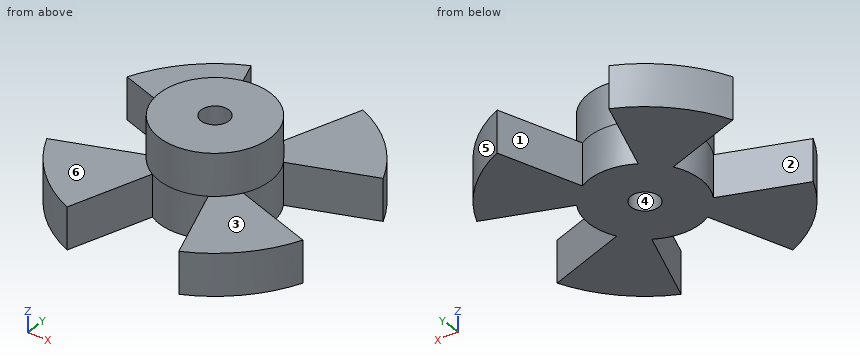
Autodesk Inventor part; units mm, degrees
ref_plane "YZ Plane" through (0, 0, 0) normal (1, 0, 0) x (0, 1, 0)
ref_plane "XZ Plane" through (0, 0, 0) normal (0, 1, 0) x (-1, 0, 0)
ref_plane "XY Plane" through (0, 0, 0) normal (0, 0, 1) x (1, 0, 0)
sketch "Esquisse1" plane through (0, 0, 0) normal (0, 0, 1) x (1, 0, 0)
  circle A0 centre (0, 0) radius 5
  dimension "d0" = 10
extrude "Extrusion1" add sketch "Esquisse1" along normal blind 1.5
sketch "Esquisse2" plane through (0, 0, 1.5) normal (0, 0, 1) x (1, 0, 0)
  circle A0 centre (0, 0) radius 5
  circle A1 centre (0, 0) radius 2
  dimension "d3" = 4
extrude "Extrusion2" add sketch "Esquisse2" along normal blind 1.5 contours A1
sketch "Esquisse3" plane through (0, 0, 1.5) normal (0, 0, 1) x (1, 0, 0)
  circle A0 centre (0, 0) radius 2
  circle A1 centre (0, 0) radius 5
  line L0 (-2, 4.5826) -> (-1, 1.7321)
  line L1 (1, 1.7321) -> (2, 4.5826)
  arc A2 (1, 1.7321) -> (-1, 1.7321) centre (0, 0) ccw
  arc A3 (2, 4.5826) -> (-2, 4.5826) centre (0, 0) ccw
extrude "Extrusion3" cut sketch "Esquisse3" against normal through all contours A0 L0 A1 L1 picked at (1.2132, 3.7931)
pattern_circular "Réseau circulaire1" count 4 over 360 about axis through (0, 0, 1.5) along (0, 0, 1) of "Extrusion3"
sketch "Esquisse4" plane through (0, 0, 3) normal (0, 0, 1) x (1, 0, 0)
  circle A0 centre (0, 0) radius 2
  circle A1 centre (0, 0) radius 0.5
  dimension "d11" = 1
extrude "Extrusion4" cut sketch "Esquisse4" against normal through all contours A1
properties part number "helice encodeur" material "Plastique ABS"
Read the model definition and answer for the solid it produces. Units are mm, in the model's axes. Face numbers are marked on the shaded views. A direction names the side the tool comes from. Coordinates: 2 decimals unless noted, no trailing zeros. Write each loop counter-clockwise with the first axis right and the second up, starting at its lowest first coordinate (ties: lowest second). Pieces come first, ordered by that corner, then holes. Notation, with made-up numbers: (-22, 86) - (9, 86) arc R24 cw to (9, 121) - close; hole circle Ø2 at (50, -34.75). An arc over 180 degrees is marked (long way). One line per question, with ' | ' between items.
Q1. Each of these flat-tipped pins is pushed along its axis until it touches: P1, Ø3, axis at x = -2.5, y = -2.5, coming from the +Z side; P2, Ø1, axis at y = 0.5, z = 2, coming from the -X side. Where does it stop, or does it pass through?
Result set:
P1: z = 1.5 | P2: x = -2
Q2. Find section A-A, the plane y = 0. Write down the section's boundary in (x, z), plus the area to 3 significant figures.
Result set:
outline: (-2, 0) - (-0.5, 0) - (-0.5, 3) - (-2, 3) - close; (0.5, 0) - (2, 0) - (2, 3) - (0.5, 3) - close | area: 9.00 mm^2
Q3. For the marked faces 1, 2 and 3, determine the directions among +Z, -Z, +X, -X, +Y, -Y from which every point of the face is accessible in a straight line to the end or side of a thin tool.
Result set:
face 1: +Z, -Z, +Y | face 2: +Z, -Z, -X | face 3: +Z, +X, -Y
Q4. Find section C-C, the plane z = 2.75. Write down the section's boundary in (x, y).
Result set:
outline: circle Ø4 at (0, 0); hole circle Ø1 at (0, 0)
Q5. Determine the mould class of the marked faces 4, 5 and 6 for opening direction Y: +Y half, -Y half, draft (parallel to the pull), parting line (faces both ways), or undercut.
Result set:
face 4: undercut | face 5: +Y half | face 6: draft
Q6. Consider L1, parallel to Y at x = 0, z = 0.9; L2, parallel to Z at x = -3, y = 3.75; L3, parallel to Y at x = -3.5, z = 0.3. Determine where each line is inside the solid, lowest interval first. Write a range as [from, to].
Result set:
L1: [-2, -0.5], [0.5, 2] | L2: [0, 1.5] | L3: [-3.57, -1.62], [1.62, 3.57]
